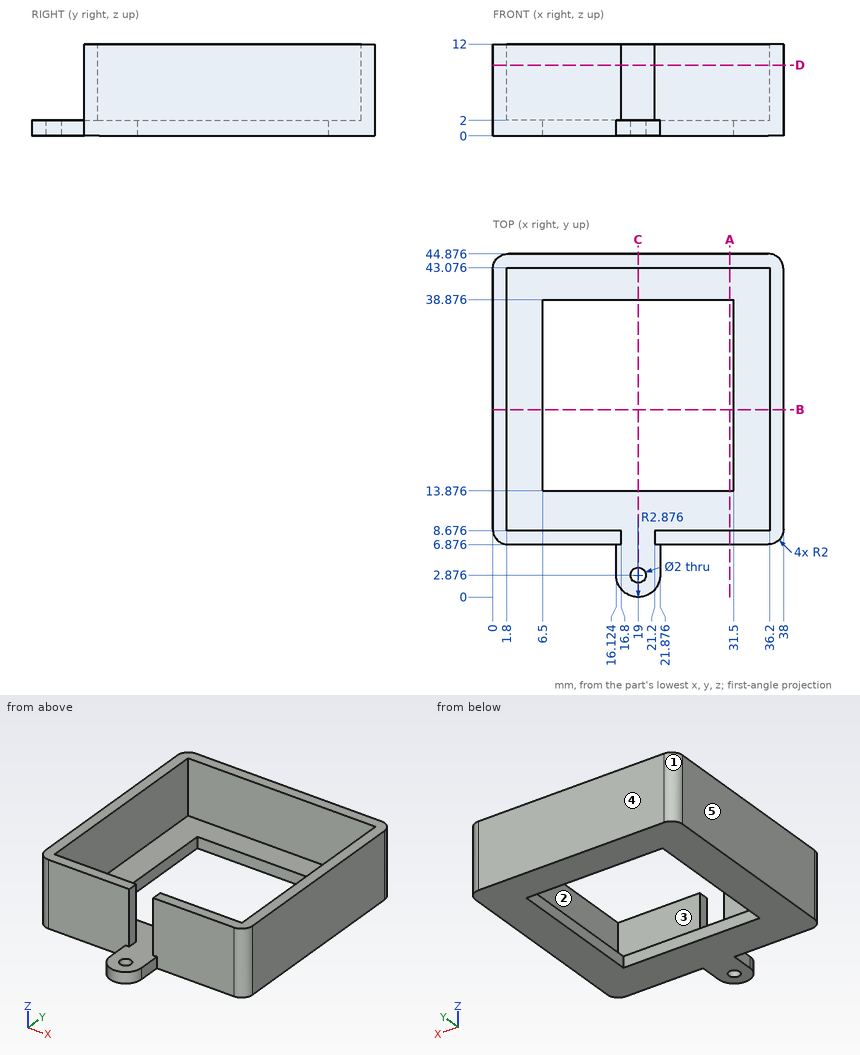
The figure shows three views and two pictorial views of one solid part (mm, origin at its lowest corner). Answer the questions. A direction names the side the tool comes from. Give positions to 0.01 mm unless a question says otherwise; leave off trailing zeros. Order: outer loops, then holes, each group sorted by start corner. A loop starts at its lowest first (then second) coordinate and runs counter-clockwise, first axis right, second up. Notation, with made-up numbers: (83, 10) -> (111, 10) arc R26 cw to (111, 29) -> close; hole circle Ø7 at (-26, 50.25). An arc over 180 degrees is marked (long way). Answer as CSV lines item,"result". Start each with the question number.
Q1. Given pin 1 (2 mm diameter, centred on y = 7.5, z = 5.5, fed in from -X); pin 2 (1 mm diameter, centred on y = 4, z = 1.5, fed in from +X); pin 3 (1 mm diameter, centred on x = 8, z = 5, fed in from -Y); pin 4 (1.6 mm diameter, centred on x = 19, y = 2.88, fed in from +Z), each flat-ended and moving along its own axis, determine where each tip first touches the part or whether it passes through.
Q2. Which of the six approach directions +Z, -Z, +X, -X, +Y, -Y give full straight-line access (tool end or side, diameter ignored) to the marked faces 1 and 2?
Q3. Determine the mould class of the marked faces 3, 4 and 5 for opening direction X: pulls with the +X half, pulls with the -X half, needs draft (parallel to the pull), parting line crosses it, or undercut.
Q4. A cutting plane is placed at B-B (y = 24.5). Determine the outline of the cut face in (x, z).
Q5. A cutting plane is placed at A-A (x = 31). Determine the outline of the cut face in (y, z).
Q6. Find the intervals of material crossed by L1, parallel to Y at x = 19, z = 1.35; L2, parallel to X at y = 39, z = 6.5; L3, parallel to Y at x = 7, z = 11.5, in increasing order.
Q7. A cutting plane is placed at C-C (x = 19). Determine the outline of the cut face in (y, z).
Q8. A cutting plane is placed at D-D (z = 9.25). Determine the outline of the cut face in (x, y).
Results found:
1,pin 1,"x = 0.04"
1,pin 2,"x = 21.88"
1,pin 3,"y = 6.88"
1,pin 4,"through"
2,face 1,"+Z, -Z, -X, +Y"
2,face 2,"+Z"
3,face 3,"undercut"
3,face 4,"needs draft"
3,face 5,"pulls with the -X half"
4,outline,"(0, 0) -> (6.5, 0) -> (6.5, 2) -> (1.8, 2) -> (1.8, 12) -> (0, 12) -> close; (31.5, 0) -> (38, 0) -> (38, 12) -> (36.2, 12) -> (36.2, 2) -> (31.5, 2) -> close"
5,outline,"(6.88, 0) -> (13.88, 0) -> (13.88, 2) -> (8.68, 2) -> (8.68, 12) -> (6.88, 12) -> close; (38.88, 0) -> (44.88, 0) -> (44.88, 12) -> (43.08, 12) -> (43.08, 2) -> (38.88, 2) -> close"
6,L1,"0 to 1.88, 3.88 to 13.88, 38.88 to 44.88"
6,L2,"0 to 1.8, 36.2 to 38"
6,L3,"6.88 to 8.68, 43.08 to 44.88"
7,outline,"(0, 0) -> (1.88, 0) -> (1.88, 2) -> (0, 2) -> close; (3.88, 0) -> (13.88, 0) -> (13.88, 2) -> (3.88, 2) -> close; (38.88, 0) -> (44.88, 0) -> (44.88, 12) -> (43.08, 12) -> (43.08, 2) -> (38.88, 2) -> close"
8,outline,"(0, 8.88) arc R2 ccw to (2, 6.88) -> (16.8, 6.88) -> (16.8, 8.68) -> (1.8, 8.68) -> (1.8, 43.08) -> (36.2, 43.08) -> (36.2, 8.68) -> (21.2, 8.68) -> (21.2, 6.88) -> (36, 6.88) arc R2 ccw to (38, 8.88) -> (38, 42.88) arc R2 ccw to (36, 44.88) -> (2, 44.88) arc R2 ccw to (0, 42.88) -> close"
